from build123d import *

# Parameters (mm, degrees)
SZKIC1_R = 2.5


with BuildPart() as part:
    # Wyciągnięcie po ścieżce1: sweep along a path in Szkic2
    with BuildLine(Plane.XY) as wyci_gni_cie_po_cie_ce1_path:
        Line((20.821502931, -29.975890373), (12.185665565, -22.729562424))
        ThreePointArc((12.185665565, -22.729562424), (8.146437857, -16.389244949), (8.474352926, -8.878755094))
        Line((8.474352926, -8.878755094), (10.77231686, -2.565151075))
        ThreePointArc((10.77231686, -2.565151075), (11.224622204, 0), (10.77231686, 2.565151075))
        Line((10.77231686, 2.565151075), (8.474352926, 8.878755094))
        ThreePointArc((8.474352926, 8.878755094), (8.146437857, 16.389244949), (12.185665565, 22.729562424))
        Line((12.185665565, 22.729562424), (23.892544244, 32.552800006))
        ThreePointArc((23.892544244, 32.552800006), (25.078385042, 34.098217822), (25.5, 36))
        ThreePointArc((25.5, 36), (14, 47.5), (2.5, 36))
        Line((2.5, 36), (2.5, -52.5))
    # Szkic1 → Wyciągnięcie po ścieżce1 (sweep)
    with BuildSketch(Plane(origin=(0, -52.5, 0), x_dir=(1, 0, 0), z_dir=(0, 1, 0))):
        Circle(SZKIC1_R)
    sweep(path=wyci_gni_cie_po_cie_ce1_path.line)


solid = part.part
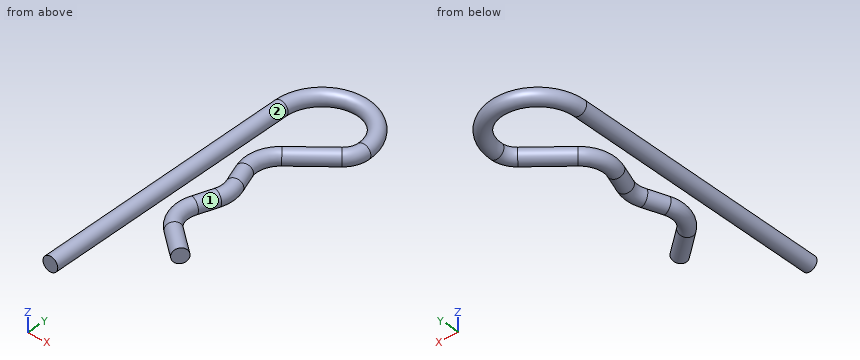
Here's how the part is built. I have some questions about the finished solid (model axes, mm). Face numbers are marked on the shaded views. A direction names the side the tool comes from. Round coordinates to 2 decimals unless told otherwise and drop trailing zeros. Order: outer loops, then holes, each group sorted by start corner. A loop starts at its lowest first (then second) coordinate and runs counter-clockwise, first axis right, second up. Notation, with made-up numbers: (41.5, 41) -> (96.5, 41) arc R7 cw to (96.5, 51) -> close; hole circle Ø8 at (33.5, 47.25). An arc over 180 degrees is marked (long way). Return JSON: item names as keys, results as strings.
Q1. For pin 1 Ø1.5 at (y, z) = (-34.5, 0.5) entering from +X; pin 2 Ø6 at (x, y) = (15, -27.5) entering from -Z; pin 3 Ø4 at (x, y) = (8.5, -18.5) entering from +Z, each with a flat end and sliding along its axis, tell me the tip position at first contact or that it passes through.
Filled sheet:
{"pin 1": "stops at x = 2.5", "pin 2": "stops at z = -2.11", "pin 3": "stops at z = 2.34"}
Q2. I need wall thicknesses on line 1 along Y through (x, z) = (20, 0.85); line 2 along Y through (x, z) = (23.5, 0.55); line 3 along Y through (x, z) = (24, 1.4). Which ranges of each line are inside material? Lowest first, please. Write a range as from..to.
Filled sheet:
{"line 1": "y = -29.09..-22.95, 22.95..29.09, 45.98..51.21", "line 2": "y = -26.78..-25.78, 25.78..32.14, 42.59..49.42", "line 3": "y = 26.68..32.08, 42.5..48.58"}
Q3. If we section it at B-B on y = -35.5: List the corners of the cut face in (x, z) for me.
Filled sheet:
{"outline": "circle Ø5 at (0, 0)"}
Q4. If we section it at A-A on z = 1.15: List the corners of the cut face in (x, y) for me, plus the area to 3 significant figures.
Filled sheet:
{"outline": "(-2.22, -52.5) -> (2.22, -52.5) -> (2.22, 36) arc R11.78 cw to (25.78, 36) arc R4.78 cw to (24.07, 32.34) -> (12.37, 22.51) arc R12.22 ccw to (8.74, 8.97) -> (11.04, 2.66) arc R7.78 cw to (11.04, -2.66) -> (8.74, -8.97) arc R12.22 ccw to (12.37, -22.51) -> (21, -29.76) -> (23.86, -26.36) -> (15.22, -19.11) arc R7.78 cw to (12.91, -10.49) -> (15.21, -4.18) arc R12.22 ccw to (15.21, 4.18) -> (12.91, 10.49) arc R7.78 cw to (15.22, 19.11) -> (26.93, 28.94) arc R9.22 ccw to (30.22, 36) arc R16.22 ccw to (-2.22, 36) -> close", "area": "932 mm^2"}
Q5. Which directions (+Z, -Z, +X, -X, +Y, -Y) give clear straight access to the entire face, cutting with the end or side of a thin tool? Please do the marked faces 1 and 2.
Filled sheet:
{"face 1": "none", "face 2": "-Y"}
